The model under review builds one solid part; all positions refer to its coordinate system, in mm. A direction names the side the tool comes from. Coordinates: 2 decimals unless noted, no trailing zeros. Loops run counter-clockwise (first coordinate to the right, second up) from the corner with the lowest first, then second, coordinate; pieces in that order, holes last. Notation, with made-up numbers: (72, -32) - (80, -32) arc R25 cw to (80, -9) - close; hole circle Ø11 at (-14.75, 15). An arc over 180 degrees is marked (long way). Answer in a Markdown table with one row per item. Add a question column.
(1) We need section A-A on y = 0. Write out the cut boundary in (x, z), plus the area to 3 significant figures.
(2) Machinability: for faces 1 (the flat face through (2, -13, 0)), 2 (the flat face through (0, 6, -2)), 3 (the cylindrical face through (-12.5, -0.1, -5)), which of the approach directions +Z, -Z, +X, -X, +Y, -Y give a long, thin tool a straight path to every point of the face, cutting with its end or side? Answer none if there is none.
(3) For line 1 along Y through (x, z) = (0, -7); line 2 along Y through (x, z) = (15.05, -5.7); line 3 along Z through (x, y) = (-15.5, 5), list the stretches that pass through material, from the lowest coordinate up.
(4) We need section C-C on z = -6. Give the number of separate pieces and of enclosed holes in the cut face, plus the area to 3 significant figures.
(5) Mouldability with a two-part tool opening along Y and no side actions: class faces 4 (the cylindrical face through (-5.506, -24.796, -3.944)), 5 (the flat face through (0, 5, -5)), 6 (the flat face through (-0.4, -5.3, -8)) as +Y half, -Y half, draft (parallel to the pull), parting line (faces both ways), or undercut.
(6) For P1, Ø4, axis at x = -15.05, y = -8.5, coming from the +Z side; P2, Ø3.5, axis at y = -18, z = -3, coming from the +X side; P3, Ø4, axis at x = -2.5, z = -5, coming from the -Y side, all flat-tipped, find the tip position at first contact; note any pin that passes through.
(7) We need section B-B on x = 0. Write out the cut boundary in (y, z).
from build123d import *

# Parameters (mm, degrees)
SKETCH1_R             = 25.4
BOSS_EXTRUDE1_DEPTH   = 8
CUT_EXTRUDE1_DEPTH    = 2
CUT_EXTRUDE2_DEPTH    = 37.418676527
F_8_32_TAPPED_HOLE1_D = 3.4544
CUT_EXTRUDE3_DEPTH    = 37.80108694
SKETCH7_W             = 19.05
SKETCH7_H             = 6
CUT_EXTRUDE4_DEPTH    = 37.80108694
FILLET1_R             = 1.5


with BuildPart() as part:
    # Sketch1 → Boss-Extrude1 (new body)
    with BuildSketch(Plane.XY):
        Circle(SKETCH1_R)
    extrude(amount=-BOSS_EXTRUDE1_DEPTH)

    # Sketch2 → Cut-Extrude1 (cut)
    with BuildSketch(Plane.XY):
        with BuildLine():
            Line((-16.55, 12.5), (16.55, 12.5))
            ThreePointArc((16.55, 12.5), (18.317766953, 11.767766953), (19.05, 10))
            Line((19.05, 10), (19.05, -10))
            ThreePointArc((19.05, -10), (18.317766953, -11.767766953), (16.55, -12.5))
            Line((16.55, -12.5), (-16.55, -12.5))
            ThreePointArc((-16.55, -12.5), (-18.317766953, -11.767766953), (-19.05, -10))
            Line((-19.05, -10), (-19.05, 10))
            ThreePointArc((-19.05, 10), (-18.317766953, 11.767766953), (-16.55, 12.5))
        make_face()
    extrude(amount=-CUT_EXTRUDE1_DEPTH, mode=Mode.SUBTRACT)

    # Sketch3 → Cut-Extrude2 (cut, through all)
    with BuildSketch(Plane.XY.offset(-2)):
        with BuildLine():
            Line((-7.5, 5), (7.5, 5))
            ThreePointArc((7.5, 5), (12.5, 0), (7.5, -5))
            Line((7.5, -5), (-7.5, -5))
            ThreePointArc((-7.5, -5), (-12.5, 0), (-7.5, 5))
        make_face()
    extrude(amount=-CUT_EXTRUDE2_DEPTH, mode=Mode.SUBTRACT)

    # #8-32 Tapped Hole1 (through all)
    with Locations(Plane.XY.offset(-2)):
        with Locations((15.05, 8.5), (-15.05, 8.5), (-15.05, -8.5), (15.05, -8.5)):
            Hole(F_8_32_TAPPED_HOLE1_D / 2)

    # Sketch6 → Cut-Extrude3 (cut, through all)
    with BuildSketch(Plane.XY):
        with BuildLine():
            Line((6.4375, 21.75), (-6.4375, 21.75))
            ThreePointArc((-6.4375, 21.75), (-7.498160172, 21.310660172), (-7.9375, 20.25))
            Line((-7.9375, 20.25), (-7.9375, 15.75))
            ThreePointArc((-7.9375, 15.75), (-7.498160172, 14.689339828), (-6.4375, 14.25))
            Line((-6.4375, 14.25), (6.4375, 14.25))
            ThreePointArc((6.4375, 14.25), (7.498160172, 14.689339828), (7.9375, 15.75))
            Line((7.9375, 15.75), (7.9375, 20.25))
            ThreePointArc((7.9375, 20.25), (7.498160172, 21.310660172), (6.4375, 21.75))
        make_face()
    extrude(amount=-CUT_EXTRUDE3_DEPTH, mode=Mode.SUBTRACT)

    # Sketch7 → Cut-Extrude4 (cut, through all)
    with BuildSketch(Plane.XY):
        with Locations((0, -18)):
            Rectangle(SKETCH7_W, SKETCH7_H)
    extrude(amount=-CUT_EXTRUDE4_DEPTH, mode=Mode.SUBTRACT)

    # Fillet1
    fillet1_edges = [part.edges().sort_by_distance(p)[0] for p in [
        (9.525, -15, -4),
        (9.525, -21, -4),
        (-9.525, -21, -4),
        (-9.525, -15, -4),
    ]]
    fillet(fillet1_edges, radius=FILLET1_R)


solid = part.part
Outcome:
| question | item | result |
|---|---|---|
| 1 | outline | (-25.4, -8) - (-12.5, -8) - (-12.5, -2) - (-19.05, -2) - (-19.05, 0) - (-25.4, 0) - close; (12.5, -8) - (25.4, -8) - (25.4, 0) - (19.05, 0) - (19.05, -2) - (12.5, -2) - close |
| 1 | area | 180 mm² |
| 2 | face 1 | +Z, +X, -X, +Y, -Y |
| 2 | face 2 | +Z |
| 2 | face 3 | +Z, -Z |
| 3 | line 1 | -25.4 to -21, -15 to -5, 5 to 14.25, 21.75 to 25.4 |
| 3 | line 2 | -20.46 to -10.23, -6.77 to 6.77, 10.23 to 20.46 |
| 3 | line 3 | -8 to -2 |
| 4 | separate pieces | 1 |
| 4 | enclosed holes | 7 |
| 4 | area | 1,530 mm² |
| 5 | face 4 | parting line |
| 5 | face 5 | undercut |
| 5 | face 6 | draft |
| 6 | P1 | z = -2 |
| 6 | P2 | x = 19.52 |
| 6 | P3 | y = -25.4 |
| 7 | outline | (-25.4, -8) - (-21, -8) - (-21, 0) - (-25.4, 0) - close; (-15, -8) - (-5, -8) - (-5, -2) - (-12.5, -2) - (-12.5, 0) - (-15, 0) - close; (5, -8) - (14.25, -8) - (14.25, 0) - (12.5, 0) - (12.5, -2) - (5, -2) - close; (21.75, -8) - (25.4, -8) - (25.4, 0) - (21.75, 0) - close |
